from build123d import *

# Parameters (mm, degrees)
SKETCH1_R          = 5
BASE_EXTRUDE_DEPTH = 15
CUT_EXTRUDE1_DEPTH = 5


with BuildPart() as part:
    # Sketch1 → Base-Extrude (new, symmetric)
    with BuildSketch(Plane.XY):
        with BuildLine():
            Line((30.426111358, 20.139143504), (19.180390516, -15.739203845))
            ThreePointArc((19.180390516, -15.739203845), (0.542906018, -29.514464646), (-18.256979683, -15.96168131))
            Line((-18.256979683, -15.96168131), (-30, 20))
            Line((-30, 20), (-50, 20))
            Line((-50, 20), (-50, 40))
            Line((-50, 40), (50.426111358, 40))
            Line((50.426111358, 40), (50.426111358, 20.139143504))
            Line((50.426111358, 20.139143504), (30.426111358, 20.139143504))
        make_face()
        with Locations((0.426111358, -9.860856496)):
            Circle(SKETCH1_R, mode=Mode.SUBTRACT)
    extrude(amount=BASE_EXTRUDE_DEPTH, both=True)

    # Sketch2 → Cut-Extrude1 (cut, symmetric)
    with BuildSketch(Plane.XY):
        with BuildLine():
            Line((-50.148365525, -40), (50.000039492, -40))
            Line((50.000039492, -40), (6.45662049, -2.46739488))
            ThreePointArc((6.45662049, -2.46739488), (-0.072081984, -0.041909569), (-6.600887406, -2.467117756))
            Line((-6.600887406, -2.467117756), (-50.148365525, -40))
        make_face()
    extrude(amount=CUT_EXTRUDE1_DEPTH, both=True, mode=Mode.SUBTRACT)


solid = part.part
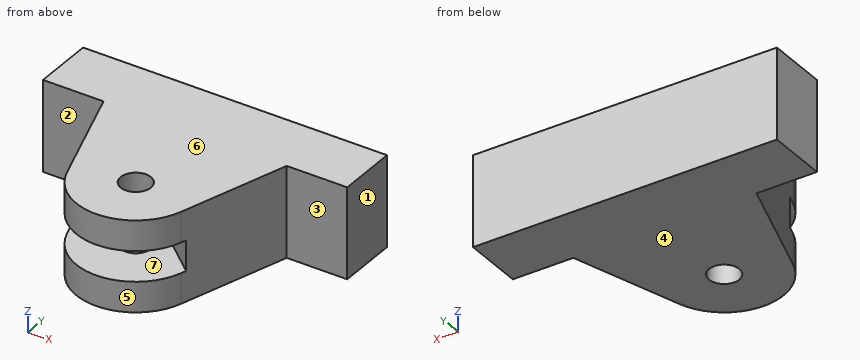
For this review, take the finished solid that the model builds, in its own axes (mm). Face numbers are marked on the shaded views. A direction names the side the tool comes from. Round coordinates to 2 decimals unless told otherwise and drop trailing zeros. Write each loop counter-clockwise with the first axis right and the second up, starting at its lowest first coordinate (ties: lowest second). Pieces come first, ordered by that corner, then holes. Notation, with made-up numbers: M 0,18.5 L 47,18.5 A16 cw 47,42.5 Z; hole C 67.5,53 d11. An arc over 180 degrees is marked long. Write item = value, one per line. Start each with the question number.
(1) The part is to be moulded in two halves that separate along Z. For the marked faces 4, 5, 6 and 7, say which applies: +Z half, -Z half, draft (parallel to the pull), parting line (faces both ways), or undercut.
(2) Clearance check with flat-ended pins moving along their axes: pin 1 Ø3 at (y, z) = (-1.5, -10) entering from -X; pin 2 Ø6 at (x, z) = (-42, 3) entering from -Y. State where each tip first meets the part, or that it passes through.
(3) We need section C-C (z = 10). Give the boundary of the cut face in (x, y), then the cut area to 3 significant figures.
(4) For line 1 along Y through (x, z) = (45, -13.25); line 2 along Z through (x, y) = (13.5, -14); line 3 along X through (y, z) = (-7.5, 2), list the stretches that pass through material, from the lowest coordinate up.
(5) We need section B-B (y = -8.5). Give the boundary of the cut face in (x, z), then the cut area to 3 significant figures.
(6) We need section D-D (x = -2). Give the boundary of the cut face in (y, z).
(7) We need section A-A (z = -3). Give the boundary of the cut face in (x, y), then the cut area to 3 significant figures.
(8) For the marked faces 1, 2 and 3, list the 3-axis set-ups (+Z, -Z, +X, -X, +Y, -Y) from which the entire face can be reached by the end or side of a thin tool; tool diameter is ignored.
Results found:
q1.face_4 = -Z half
q1.face_5 = draft
q1.face_6 = +Z half
q1.face_7 = undercut
q2.pin_1 = -23.47
q2.pin_2 = 20
q3.outline = M -50,20 L -30,20 L -18.26,-15.96 A19.65 ccw 19.18,-15.74 L 30.43,20.14 L 50.43,20.14 L 50.43,40 L -50,40 Z; hole C 0.43,-9.86 d10
q3.area = 4,060 mm²
q4.line_1 = 20.14 to 40
q4.line_2 = -15 to -5, 5 to 15
q4.line_3 = -21.02 to -12.44, 12.3 to 21.76
q5.outline = M -20.69,-15 L -4.39,-15 L -4.39,-5 L -13.6,-5 L -13.6,5 L -4.39,5 L -4.39,15 L -20.69,15 Z; M 5.24,-15 L 21.45,-15 L 21.45,15 L 5.24,15 L 5.24,5 L 13.46,5 L 13.46,-5 L 5.24,-5 Z
q5.area = 801 mm²
q6.outline = M -29.36,-15 L -14.23,-15 L -14.23,-5 L -29.36,-5 Z; M -29.36,5 L -14.23,5 L -14.23,15 L -29.36,15 Z; M -5.49,-15 L 40,-15 L 40,15 L -5.49,15 L -5.49,5 L -0.23,5 L -0.23,-5 L -5.49,-5 Z
q7.outline = M -50,20 L -30,20 L -19.14,-13.27 L -6.6,-2.47 A10 cw 6.46,-2.47 L 19.75,-13.92 L 30.43,20.14 L 50.43,20.14 L 50.43,40 L -50,40 Z
q7.area = 3,360 mm²
q8.face_1 = +Z, -Z, +X, +Y, -Y
q8.face_2 = +Z, -Z, -X, -Y
q8.face_3 = +Z, -Z, +X, -Y
